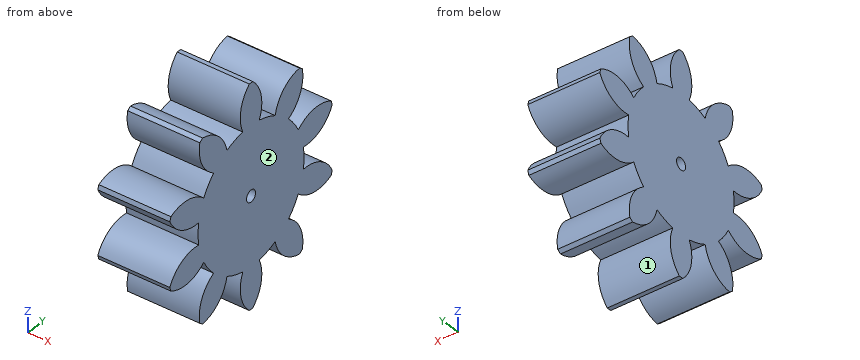
```python
from build123d import *

# Parameters (mm, degrees)
BASPROSKE_W              = 12
BASPROSKE_H              = 7.5
TOOTHCUT_DEPTH           = 17.015617378
TEETHCUTS_COUNT          = 10
TEETHCUTS_ANGLE          = 324
BORSKE_R                 = 0.4
BORE_DEPTH               = 50.0000508
SCHIZZO1_W               = 18.724630976
SCHIZZO1_H               = 16.705622174
TAGLIO_ESTRUSIONE1_DEPTH = 7


with BuildPart() as part:
    # BasProSke → Base-Revolve (revolve)
    with BuildSketch(Plane(origin=(0, 0, 0), x_dir=(1, 0, 0), z_dir=(0, 1, 0)), mode=Mode.PRIVATE) as base_revolve_sk:
        with Locations((6, 3.75)):
            Rectangle(BASPROSKE_W, BASPROSKE_H)
    revolve(base_revolve_sk.sketch.rotate(Axis((-10, 0, 0), (1, 0, 0)), 180), axis=Axis((-10, 0, 0), (1, 0, 0)))

    # TooCutSke → ToothCut (cut, through all)
    with BuildSketch(Plane(origin=(0, 0, 0), x_dir=(0, 0, -1), z_dir=(1, 0, 0))):
        with BuildLine():
            ThreePointArc((0.737676151, 4.628079099), (0, 4.6865), (-0.737676151, 4.628079099))
            ThreePointArc((-0.737676151, 4.628079099), (-1.051542781, 6.151798382), (-2.205760267, 7.194877817))
            ThreePointArc((-2.205760267, 7.194877817), (0, 7.5254), (2.205760267, 7.194877817))
            ThreePointArc((2.205760267, 7.194877817), (1.051542781, 6.151798382), (0.737676151, 4.628079099))
        make_face()
    toothcut = extrude(amount=TOOTHCUT_DEPTH, mode=Mode.SUBTRACT)

    # TeethCuts: ToothCut ×10 about axis
    teethcuts_axis = Axis((-10, 0, 0), (1, 0, 0))
    for i in range(1, TEETHCUTS_COUNT):
        add(toothcut.rotate(teethcuts_axis, i * TEETHCUTS_ANGLE / (TEETHCUTS_COUNT - 1)), mode=Mode.SUBTRACT)

    # BorSke → Bore (cut, symmetric)
    with BuildSketch(Plane(origin=(0, 0, 0), x_dir=(0, 0, -1), z_dir=(1, 0, 0))):
        with Locations(Location((0, 0, 0), (0, 0, 180))):
            Circle(BORSKE_R)
    extrude(amount=BORE_DEPTH, both=True, mode=Mode.SUBTRACT)

    # Schizzo1 → Taglio-Estrusione1 (cut)
    with BuildSketch(Plane(origin=(12, 0, 0), x_dir=(0, 0, -1), z_dir=(1, 0, 0))):
        Rectangle(SCHIZZO1_W, SCHIZZO1_H)
    extrude(amount=-TAGLIO_ESTRUSIONE1_DEPTH, mode=Mode.SUBTRACT)


solid = part.part
```
Design review of the part built by this model. Coordinates are the model's own, in mm. Face numbers are marked on the shaded views. Give positions to 0.01 mm unless a question says otherwise; leave off trailing zeros. Write each loop counter-clockwise with the first axis right and the second up, starting at its lowest first coordinate (ties: lowest second). Pieces come first, ordered by that corner, then holes. Notation, with made-up numbers: (-27, -34) -> (32, -34) arc R16 ccw to (32, -7) -> close; hole circle Ø1 at (-6.75, 82.25). An arc over 180 degrees is marked (long way). Answer in a Markdown table with one row per item.
(1) Mouldability with a two-part tool opening along Y and no side actions: class the marked faces 1 and 2 as +Y half, -Y half, draft (parallel to the pull), parting line (faces both ways), or undercut.
Results:
| item | result |
|---|---|
| face 1 | undercut |
| face 2 | draft |
(2) Consider section C-C (y = -1.5). State the section outline as (x, z) points, then the cut area to 3 significant figures.
Results:
| item | result |
|---|---|
| outline | (0, -4.44) -> (5, -4.44) -> (5, 4.44) -> (0, 4.44) -> close |
| area | 44.4 mm2 |
(3) Consider section A-A (z = 0). State the section outline as (x, y) points.
Results:
| item | result |
|---|---|
| outline | (0, -4.69) -> (5, -4.69) -> (5, -0.4) -> (0, -0.4) -> close; (0, 0.4) -> (5, 0.4) -> (5, 4.69) -> (0, 4.69) -> close |
(4) Clearance check with flat-ended pins moving along their axes: pin 1 (3 mm diameter, centred on x = 1.5, z = -4, fed in from +Y); pin 2 (1 mm diameter, centred on x = 3.5, z = 5, fed in from +Y). State where each tip first meets the part, or that it passes through.
Results:
| item | result |
|---|---|
| pin 1 | y = 7.02 |
| pin 2 | y = 4.58 |
(5) To check wall thickness, follow probe 1 along Y at (x, z) = (2.2, 0); probe 2 along Y at (x, z) = (1.95, 5.5); probe 3 along Z at (x, y) = (1.4, 4). State the ranges of each line that lie inside material, in increasing order.
Results:
| item | result |
|---|---|
| probe 1 | -4.69 to -0.4, 0.4 to 4.69 |
| probe 2 | -4.58 to -2.87, -0.95 to 0.95, 2.87 to 4.58 |
| probe 3 | -6.11 to -3.89, -2.44 to 2.44, 3.89 to 6.11 |
(6) Consider section B-B (z = 5). State the section outline as (x, y) points, then the cut area to 3 significant figures.
Results:
| item | result |
|---|---|
| outline | (0, -4.53) -> (5, -4.53) -> (5, -2.46) -> (0, -2.46) -> close; (0, -0.86) -> (5, -0.86) -> (5, 0.86) -> (0, 0.86) -> close; (0, 2.46) -> (5, 2.46) -> (5, 4.53) -> (0, 4.53) -> close |
| area | 29.3 mm2 |
